from build123d import *

# Parameters (mm, degrees)
EXTRUDE_1_DEPTH     = 19
SKETCH_2_R          = 3
CUT_EXTRUDE_1_DEPTH = 19
SKETCH_3_R          = 3
CUT_EXTRUDE_2_DEPTH = 19


with BuildPart() as part:
    # 草图1 → 凸台-拉伸1 (new body)
    with BuildSketch(Plane.XY):
        Polygon((0, 0), (31, 0), (31, 31), (29, 31), (29, 2), (0, 2), align=None)
    extrude(amount=EXTRUDE_1_DEPTH)

    # 草图2 → 切除-拉伸1 (cut)
    with BuildSketch(Plane.ZY.offset(-29)):
        with Locations(Location((7.709838353, 11, 0), (0, 0, 270))):
            Circle(SKETCH_2_R)
        with Locations(Location((12.709838353, 23, 0), (0, 0, 270))):
            Circle(SKETCH_2_R)
    extrude(amount=-CUT_EXTRUDE_1_DEPTH, mode=Mode.SUBTRACT)

    # 草图3 → 切除-拉伸2 (cut)
    with BuildSketch(Plane(origin=(0, 2, 0), x_dir=(1, 0, 0), z_dir=(0, 1, 0))):
        with Locations(Location((20, -8.156857101, 0), (0, 0, 180))):
            Circle(SKETCH_3_R)
        with Locations(Location((8, -13.156857101, 0), (0, 0, 180))):
            Circle(SKETCH_3_R)
    extrude(amount=-CUT_EXTRUDE_2_DEPTH, mode=Mode.SUBTRACT)


solid = part.part
The listing builds one solid part. Answer for the finished solid, in the listing's coordinates (mm). A direction names the side the tool comes from. Round coordinates to 2 decimals unless told otherwise and drop trailing zeros. Write each loop counter-clockwise with the first axis right and the second up, starting at its lowest first coordinate (ties: lowest second). Pieces come first, ordered by that corner, then holes. Notation, with made-up numbers: M 57,13.25 L 114,13.25 A14 cw 114,38.25 Z; hole C 7.25,24.25 d1. An arc over 180 degrees is marked long. Write each question's results on one line, items separated by ' | '. Start each with the question number.
Item 1: Find section A-A on y = 11. Write down the section's boundary in (x, z), and give its area (3 significant figures).
Item 2: Which of the six approach directions +Z, -Z, +X, -X, +Y, -Y give full straight-line access (tool end or side, diameter ignored) to faces 4 (the flat face through (15, 2, 9)), 5 (the flat face through (0, 1, 9))?
Item 3: Find section B-B on x = 20. Write down the section's boundary in (y, z), and give its area (3 significant figures).
Item 4: Find section D-D on x = 14.5. Write down the section's boundary in (y, z), and give its area (3 significant figures).
Item 5: Find section C-C on z = 17. Write down the section's boundary in (x, y).
Item 6: The mould has two halves that part along Y. Classify faces 1 (the flat face through (29, 17, 9)), 2 (the flat face through (30, 31, 9)), 3 (the cylindrical face through (29.99, 13.21, 9.74)): +Y half, -Y half, draft (parallel to the pull), parting line (faces both ways), or undercut.
Item 7: Straight lines are drawn through the part: probe 1 along Z at (x, y) = (30.2, 11); probe 2 along Z at (x, y) = (20, 1); probe 3 along Y at (x, z) = (12, 13.5). For each, find the intervals that lie inside material, in ascending order.
Item 8: Given pin 1 Ø3 at (x, z) = (19, 6.5) entering from +Y; pin 2 Ø4 at (x, y) = (4, 4.5) entering from -Z; pin 3 Ø5.5 at (y, z) = (20.5, 8.5) entering from -X, each flat-ended and moving along its own axis, determine where each tip first touches the part or whether it passes through.
Answer block:
1) outline: M 29,0 L 31,0 L 31,4.71 L 29,4.71 Z; M 29,10.71 L 31,10.71 L 31,19 L 29,19 Z | area: 26.0 mm²
2) face 4: +Z, -Z, -X, +Y | face 5: +Z, -Z, -X, +Y, -Y
3) outline: M 0,0 L 2,0 L 2,5.16 L 0,5.16 Z; M 0,11.16 L 2,11.16 L 2,19 L 0,19 Z | area: 26.0 mm²
4) outline: M 0,0 L 2,0 L 2,19 L 0,19 Z | area: 38.0 mm²
5) outline: M 0,0 L 31,0 L 31,31 L 29,31 L 29,2 L 0,2 Z
6) face 1: draft | face 2: +Y half | face 3: undercut
7) probe 1: z = 0 to 4.71, 10.71 to 19 | probe 2: z = 0 to 5.16, 11.16 to 19 | probe 3: y = 0 to 2
8) pin 1: stops at y = 2 | pin 2: passes through | pin 3: stops at x = 29
